Geometry check sheet. Reference: drawing and pictorial views, mm from the part's lowest x, y, z. A direction names the side the tool comes from. Round coordinates to 2 decimals unless told otherwise and drop trailing zeros. Loops run counter-clockwise (first coordinate to the right, second up) from the corner with the lowest first, then second, coordinate; pieces in that order, holes last. Notation, with made-up numbers: (50, -17.5) - (106, -17.5) arc R22 ccw to (106, 0.5) - close; hole circle Ø1 at (-37.5, -24). An arc over 180 degrees is marked (long way). Put each result on its own line as item: value. Start each with the question number.
Item 1: Material ranges on line 1 along X through (y, z) = (52.5, 7.75); line 2 along Z through (x, y) = (9.5, 75); line 3 along Y through (x, z) = (52, 14.5), recorded low to high.
Item 2: Tool access check on the marked faces 1 and 2. Record the directions out of +Z, -Z, +X, -X, +Y, -Y that give a thin tool (end or side, any length) a straight path to the whole face; none if there is none.
Item 3: Section check A-A, the plane y = 35. Record the cut outline in (x, z), and give its area (3 significant figures).
Item 4: Section check B-B, the plane x = 28.5. Record the cut outline in (y, z), and give its area (3 significant figures).
Item 5: Draft check along Y on the marked faces 3, 4, 5 and 6. Enter one of: pulls with the +Y half, pulls with the -Y half, needs draft (parallel to the pull), parting line crosses it, or undercut.
Item 6: Gauge pin test, flat ends, axial feed: pin 1 Ø10 at (x, y) = (12.625, 47.625) entering from +Z (1 decimal); pin 2 Ø1.5 at (y, z) = (30.5, 11) entering from -X; pin 3 Ø10 at (x, z) = (42, 3) entering from +Y. Record the tip position at first contact, or that the pin passes through.
Item 7: Section check C-C, the plane y = 66. Record the cut outline in (x, z), and give its area (3 significant figures).
Item 8: Section check D-D, the plane z = 15.5. Record the cut outline in (x, y) (3 decimals), and give its area (3 significant figures).
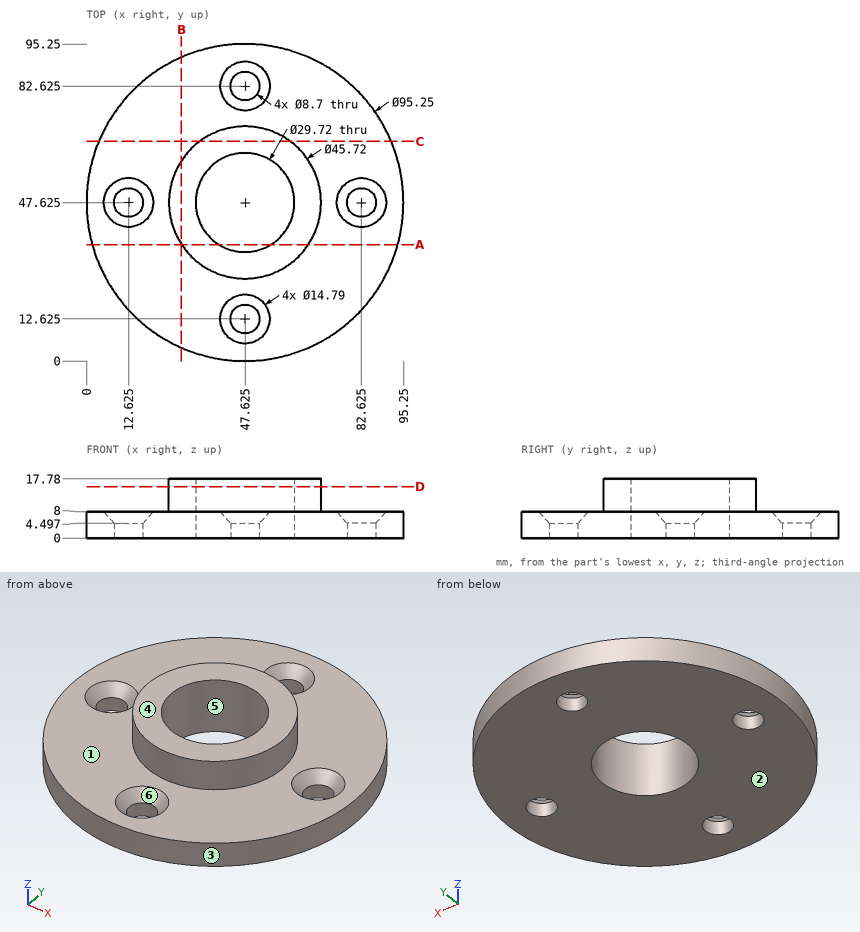
Check result:
1. line 1: 0.25 to 7.36, 17.89 to 33.59, 61.66 to 77.36, 87.89 to 95
1. line 2: 0 to 8
1. line 3: 25.19 to 33.42, 61.83 to 70.06
2. face 1: +Z
2. face 2: -Z, +X, -X, +Y, -Y
3. outline: (1.7, 0) - (39.79, 0) - (39.79, 17.78) - (28.57, 17.78) - (28.57, 8) - (1.7, 8) - close; (55.46, 0) - (93.55, 0) - (93.55, 8) - (66.68, 8) - (66.68, 17.78) - (55.46, 17.78) - close
3. area: 829 mm²
4. outline: (4.01, 0) - (91.24, 0) - (91.24, 8) - (60.15, 8) - (60.15, 17.78) - (35.1, 17.78) - (35.1, 8) - (4.01, 8) - close
4. area: 943 mm²
5. face 3: parting line crosses it
5. face 4: needs draft
5. face 5: undercut
5. face 6: undercut
6. pin 1: z = 5.2
6. pin 2: x = 31.67
6. pin 3: y = 95.25
7. outline: (3.69, 0) - (91.56, 0) - (91.56, 8) - (61.22, 8) - (61.22, 17.78) - (34.03, 17.78) - (34.03, 8) - (3.69, 8) - close
7. area: 969 mm²
8. outline: circle Ø45.72 at (47.625, 47.625); hole circle Ø29.72 at (47.625, 47.625)
8. area: 948 mm²
